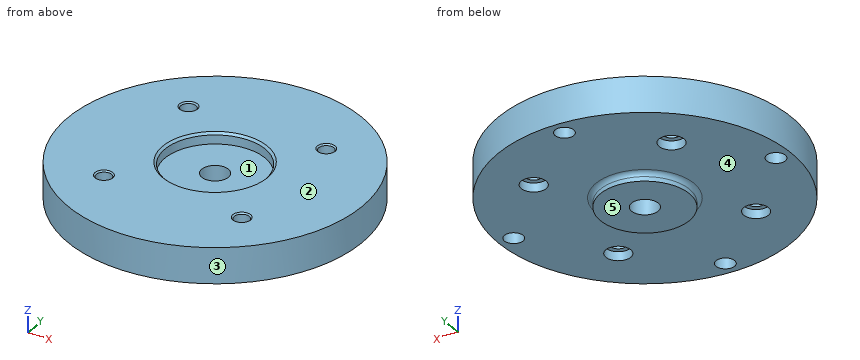
```python
from build123d import *

# Parameters (mm, degrees)
SKETCH2_R               = 33
BOSS_EXTRUDE1_DEPTH     = 8
SKETCH6_R               = 10
BOSS_EXTRUDE2_DEPTH     = 2
CUT_EXTRUDE1_DEPTH      = 48.728398255
CUT_EXTRUDE1_DEPTH_BACK = 48.728398255
SKETCH3_R               = 1.7
SKETCH3_R_2             = 3
CUT_EXTRUDE2_DEPTH      = 48.349762407
CUT_EXTRUDE2_DEPTH_BACK = 2
SKETCH4_R               = 2.8
SKETCH5_R               = 2.1
CUT_EXTRUDE3_DEPTH      = 6
FILLET1_R               = 1
SKETCH7_R               = 11.25
CUT_EXTRUDE4_DEPTH      = 2.5
CHAMFER1_SIZE           = 0.5
CHAMFER2_SIZE           = 0.3


with BuildPart() as part:
    # Sketch2 → Boss-Extrude1 (new body)
    with BuildSketch(Plane.XY):
        Circle(SKETCH2_R)
    extrude(amount=BOSS_EXTRUDE1_DEPTH)

    # Sketch6 → Boss-Extrude2 (add)
    with BuildSketch(Plane(origin=(0, 0, 0), x_dir=(-1, 0, 0), z_dir=(0, 0, -1))):
        Circle(SKETCH6_R)
    extrude(amount=BOSS_EXTRUDE2_DEPTH)

    # Sketch3 → Cut-Extrude1 (cut, two sides: drawn at the far end of the back side and taken through both)
    with BuildSketch(Plane.XY.offset(8).offset(-CUT_EXTRUDE1_DEPTH_BACK)):
        with Locations((-15.5, 15.5)):
            Circle(SKETCH3_R)
        with Locations((15.5, 15.5)):
            Circle(SKETCH3_R)
        with Locations((15.5, -15.5)):
            Circle(SKETCH3_R)
        with Locations((-15.5, -15.5)):
            Circle(SKETCH3_R)
        Circle(SKETCH3_R_2)
    extrude(amount=CUT_EXTRUDE1_DEPTH + CUT_EXTRUDE1_DEPTH_BACK, mode=Mode.SUBTRACT)

    # Sketch4 → Cut-Extrude2 (cut, two sides: drawn at the far end of the back side and taken through both)
    with BuildSketch(Plane(origin=(0, 0, 0), x_dir=(-1, 0, 0), z_dir=(0, 0, -1)).offset(-CUT_EXTRUDE2_DEPTH_BACK)):
        with Locations(Location((-15.5, 15.5, 0), (0, 0, 180))):
            Circle(SKETCH4_R)
        with Locations(Location((15.5, 15.5, 0), (0, 0, 180))):
            Circle(SKETCH4_R)
        with Locations(Location((15.5, -15.5, 0), (0, 0, 180))):
            Circle(SKETCH4_R)
        with Locations(Location((-15.5, -15.5, 0), (0, 0, 180))):
            Circle(SKETCH4_R)
    extrude(amount=CUT_EXTRUDE2_DEPTH + CUT_EXTRUDE2_DEPTH_BACK, mode=Mode.SUBTRACT)

    # Sketch5 → Cut-Extrude3 (cut)
    with BuildSketch(Plane(origin=(0, 0, 0), x_dir=(-1, 0, 0), z_dir=(0, 0, -1))):
        with Locations((0, 29.5)):
            Circle(SKETCH5_R)
        with Locations((29.5, 0)):
            Circle(SKETCH5_R)
        with Locations((0, -29.5)):
            Circle(SKETCH5_R)
        with Locations((-29.5, 0)):
            Circle(SKETCH5_R)
    extrude(amount=-CUT_EXTRUDE3_DEPTH, mode=Mode.SUBTRACT)

    # Fillet1
    fillet1_edges = [part.edges().sort_by_distance(p)[0] for p in [
        (10, 0, 0),
    ]]
    fillet(fillet1_edges, radius=FILLET1_R)

    # Sketch7 → Cut-Extrude4 (cut)
    with BuildSketch(Plane.XY.offset(8)):
        Circle(SKETCH7_R)
    extrude(amount=-CUT_EXTRUDE4_DEPTH, mode=Mode.SUBTRACT)

    # Chamfer1
    chamfer1_edges = [part.edges().sort_by_distance(p)[0] for p in [
        (-11.25, 0, 8),
    ]]
    chamfer(chamfer1_edges, length=CHAMFER1_SIZE)

    # Chamfer2
    chamfer2_edges = [part.edges().sort_by_distance(p)[0] for p in [
        (-17.2, -15.5, 8),
        (13.8, -15.5, 8),
        (13.8, 15.5, 8),
        (-17.2, 15.5, 8),
    ]]
    chamfer(chamfer2_edges, length=CHAMFER2_SIZE)


solid = part.part
```
Geometry: final body of the model. Coordinates: model frame, mm. Face numbers are marked on the shaded views. A direction names the side the tool comes from. Coordinates: 2 decimals unless noted, no trailing zeros. Order: outer loops, then holes, each group sorted by start corner. A loop starts at its lowest first (then second) coordinate and runs counter-clockwise, first axis right, second up. Notation, with made-up numbers: (-5.75, -7) - (1.25, -7) arc R11 ccw to (1.25, 10) - close; hole circle Ø11 at (-37.75, 20). An arc over 180 degrees is marked (long way). Write each question's results on one line, items separated by ' | '.
(1) Set-up query: the marked faces 4 and 5. Return all of +Z, -Z, +X, -X, +Y, -Y with unobstructed straight access to the full face (end or side cutting, diameter ignored); none if empty.
Values found:
face 4: -Z | face 5: -Z, +X, -X, +Y, -Y
(2) Section query A-A, the plane z = 1. Count the separate pieces of the cut face and the enclosed holes in it, plus the area to 3 significant figures.
Values found:
separate pieces: 1 | enclosed holes: 9 | area: 3,240 mm²
(3) Section query B-B, the plane x = 15.5. Return the cut outline in (y, z).
Values found:
outline: (-29.13, 0) - (-18.3, 0) - (-18.3, 2) - (-17.2, 2) - (-17.2, 7.7) - (-17.5, 8) - (-29.13, 8) - close; (-13.8, 2) - (-12.7, 2) - (-12.7, 0) - (12.7, 0) - (12.7, 2) - (13.8, 2) - (13.8, 7.7) - (13.5, 8) - (-13.5, 8) - (-13.8, 7.7) - close; (17.2, 2) - (18.3, 2) - (18.3, 0) - (29.13, 0) - (29.13, 8) - (17.5, 8) - (17.2, 7.7) - close
(4) First-contact query: pin 1 Ø4.5 at (x, y) = (0, 30.5) entering from -Z; pin 2 Ø1 at (y, z) = (10, 6.5) entering from +X; pin 3 Ø5 at (x, y) = (15.5, -15.5) entering from +Z; pin 4 Ø6 at (x, y) = (-7, 2.5) entering from +Z. Flat tips, straight axial feed; report the tip coordinate or a pass-through.
Values found:
pin 1: stops at z = 0 | pin 2: stops at x = 31.6 | pin 3: stops at z = 8 | pin 4: stops at z = 5.5
(5) Mould query, pull axis X, two halves, no side actions, for the marked faces 1, 2 and 3. Classes: +X half, -X half, draft (parallel to the pull), parting line (faces both ways), or undercut.
Values found:
face 1: undercut | face 2: draft | face 3: parting line
(6) Section query C-C, the plane y = 29.5. Return the cut outline in (x, z).
Values found:
outline: (-14.79, 0) - (-2.1, 0) - (-2.1, 6) - (2.1, 6) - (2.1, 0) - (14.79, 0) - (14.79, 8) - (-14.79, 8) - close
(7) Line query: line 1 (Y direction, x = 0, z = 3.2); line 2 (Y direction, x = 0, z = 6.75); line 3 (Y direction, x = 16, z = 6). Output: solid intervals per line, ascending. Write a range as [from, to].
Values found:
line 1: y = [-33, -31.6], [-27.4, -3], [3, 27.4], [31.6, 33] | line 2: y = [-33, -11.25], [11.25, 33] | line 3: y = [-28.86, -17.12], [-13.88, 13.88], [17.12, 28.86]
